Source: CAD feature listing. Evaluate the final solid. Frame: model axes, mm. A direction names the side the tool comes from. Coordinates: 2 decimals unless noted, no trailing zeros. Loops run counter-clockwise (first coordinate to the right, second up) from the corner with the lowest first, then second, coordinate; pieces in that order, holes last. Notation, with made-up numbers: M 31.5,49.25 L 78.5,49.25 A24 ccw 78.5,59.25 Z; hole C 3.25,14.5 d3. An arc over 180 degrees is marked long. One line per question, with ' | ' between items. Start each with the question number.
1. Mould query, pull axis Y, two halves, no side actions, for faces 1 (the cylindrical face through (-0.38, 4.29, 20.87)), 2 (the flat face through (0, -4.5, 17)), 3 (the flat face through (0, -1, 16.7)). Classes: pulls with the +Y half, pulls with the -Y half, needs draft (parallel to the pull), parting line crosses it, or undercut.
2. Access query for faces 4 (the flat face through (0, 23.2, 8)), 5 (the flat face through (0, 0, 20)), 6 (the flat face through (5, 1, 21.5)). Directions: +Z, -Z, +X, -X, +Y, -Y. A direction counts if a zero-diameter tool reaches every point of the face in a straight line with its end or side. Return the directions, or none.
3. Section query C-C, the plane z = 4.25. Output: boundary loops of the cut face in (x, y), and give its area (3 significant figures).
4. Pin query (flat end, axial travel): P1, Ø1.3, axis at x = -1, y = -2.5, coming from the +Z side; P2, Ø1.5, axis at x = 3.5, z = 20.5, coming from the +Y side; P3, Ø2.5, axis at x = -1.5, z = 19.5, coming from the -Y side. Return the tip coordinate at first contact, or that it passes through.
5. Section query D-D, the plane y = 5. Output: boundary loops of the cut face in (x, z), and give its area (3 significant figures).
6. Ray query, probe 1 along Y at (x, z) = (0, 17.3); probe 2 along Y at (x, z) = (0, 20.25); probe 3 along Y at (x, z) = (-4, 6). Return the intervals inside material, ascending.
7. Section query A-A, the plane y = 25.45. Output: boundary loops of the cut face in (x, z).
8. Section query B-B, the plane y = 11. Output: boundary loops of the cut face in (x, z), and give its area (3 significant figures).
```python
from build123d import *

# Parameters (mm, degrees)
F0_W     = 4.5
F0_H     = 1.5
F1_DEPTH = 6
F2_R     = 0.9
F3_DEPTH = 18.201
F5_DEPTH = 4.3
F6_R     = 1.75
F7_DEPTH = 10


with BuildPart() as f1:
    # F0 (on Right) → F1 (new body, symmetric)
    with BuildSketch(Plane.YZ):
        Polygon((23.2, 21.5), (0, 21.5), (0, 18.2), (0, 16.7), (0, 0), (23.2, 0), (23.2, 16.7), (23.2, 18.2), align=None)
        with Locations((-2.25, 17.45)):
            Rectangle(F0_W, F0_H)
        with Locations((25.45, 17.45)):
            Rectangle(F0_W, F0_H)
    extrude(amount=F1_DEPTH, both=True)

    # F2 (on face) → F3 (cut, through all)
    with BuildSketch(Plane.XY.offset(18.2)):
        with Locations((0, -2.25)):
            Circle(F2_R)
        with Locations((0, 25.45)):
            Circle(F2_R)
    extrude(amount=-F3_DEPTH, mode=Mode.SUBTRACT)

    # F4 (on face) → F5 (join)
    with BuildSketch(Plane.XY.offset(21.5)):
        with BuildLine():
            ThreePointArc((0, 0), (4.242641, 1.757359), (6, 6))
            ThreePointArc((6, 6), (0, 12), (-6, 6))
            ThreePointArc((-6, 6), (-4.242641, 1.757359), (0, 0))
        make_face()
    extrude(amount=F5_DEPTH)

    # F6 (on face) → F7 (cut)
    with BuildSketch(Plane.XY.offset(25.8)):
        with Locations((0, 6)):
            Circle(F6_R)
    extrude(amount=-F7_DEPTH, mode=Mode.SUBTRACT)


solid = f1.part
```
Taken from the geometry:
1) face 1: undercut | face 2: pulls with the -Y half | face 3: needs draft
2) face 4: -Z, +X, -X, +Y | face 5: +Z, +X, -X, -Y | face 6: +Z, +X, -Y
3) outline: M -6,0 L 6,0 L 6,23.2 L -6,23.2 Z | area: 278 mm^2
4) P1: z = 18.2 | P2: y = 23.2 | P3: y = 0
5) outline: M -6,0 L 6,0 L 6,21.5 L 5.92,21.5 L 5.92,25.8 L 1.44,25.8 L 1.44,15.8 L -1.44,15.8 L -1.44,25.8 L -5.92,25.8 L -5.92,21.5 L -6,21.5 Z | area: 280 mm^2
6) probe 1: -4.5 to -3.15, -1.35 to 4.25, 7.75 to 24.55, 26.35 to 27.7 | probe 2: 0 to 4.25, 7.75 to 23.2 | probe 3: 0 to 23.2
7) outline: M -6,16.7 L -0.9,16.7 L -0.9,18.2 L -6,18.2 Z; M 0.9,16.7 L 6,16.7 L 6,18.2 L 0.9,18.2 Z
8) outline: M -6,0 L 6,0 L 6,21.5 L 3.32,21.5 L 3.32,25.8 L -3.32,25.8 L -3.32,21.5 L -6,21.5 Z | area: 287 mm^2
